from build123d import *

# Parameters (mm, degrees)
BOSS_EXTRUDE1_DEPTH = 7
SKETCH2_R           = 2.5
CUT_EXTRUDE1_DEPTH  = 14


with BuildPart() as part:
    # Sketch1 → Boss-Extrude1 (new, symmetric)
    with BuildSketch(Plane(origin=(0, 0, 0), x_dir=(1, 0, 0), z_dir=(0, 1, 0))):
        Polygon((7, 1.5), (-7, 1.5), (-4, -1.5), (4, -1.5), align=None)
    extrude(amount=BOSS_EXTRUDE1_DEPTH, both=True)

    # Sketch2 → Cut-Extrude1 (cut)
    with BuildSketch(Plane(origin=(0, 0, -1.5), x_dir=(-1, 0, 0), z_dir=(0, 0, -1))):
        Circle(SKETCH2_R)
    extrude(amount=-CUT_EXTRUDE1_DEPTH, mode=Mode.SUBTRACT)


solid = part.part
Design review of the part built by this model. Coordinates are the model's own, in mm. Coordinates: 2 decimals unless noted, no trailing zeros. Order: outer loops, then holes, each group sorted by start corner. A loop starts at its lowest first (then second) coordinate and runs counter-clockwise, first axis right, second up. Notation, with made-up numbers: (57, 32.25) -> (113, 32.25) arc R10 cw to (113, 37.25) -> close; hole circle Ø11 at (26.25, 79.25). An arc over 180 degrees is marked (long way). Use one line per item in the form item = value. Start each with the question number.
(1) Add section D-D on y = 5. State the section outline as (x, z) points.
(2) Insertion check: pin 1 (1 mm diameter, centred on y = 5.5, z = 1, fed in from -X). The pin has a flat end and moves straight along its axis. Give the tip position at first contact, or say it passes through.
(3) For probe 1 along Y at (x, z) = (0, -0.5); probe 2 along Y at (x, z) = (-1, 0.55); probe 3 along Z at (x, y) = (-5, -6), list the stretches that pass through material, from the lowest coordinate up.
(4) The part is to be moulded in two halves that separate along X. For faces 1 (the flat face through (-5.5, 0.1, 0)), 2 (the cylindrical face through (0.54, -2.44, -0.02)), 3 (the flat face through (0, 7, 0)), say which applies: +X half, -X half, draft (parallel to the pull), parting line (faces both ways), or undercut.
(5) Add section C-C on z = 0.6. State the section outline as (x, y) points.
(6) Add section B-B on y = 0. State the section outline as (x, z) points, plus the area to 3 significant figures.
(7) Add section A-A on x = -2. State the section outline as (y, z) points, plus the area to 3 significant figures.
Answer block:
q1.outline = (-7, -1.5) -> (7, -1.5) -> (4, 1.5) -> (-4, 1.5) -> close
q2.pin_1 = -5
q3.probe_1 = -7 to -2.5, 2.5 to 7
q3.probe_2 = -7 to -2.29, 2.29 to 7
q3.probe_3 = -1.5 to 0.5
q4.face_1 = -X half
q4.face_2 = undercut
q4.face_3 = draft
q5.outline = (-4.9, -7) -> (4.9, -7) -> (4.9, 7) -> (-4.9, 7) -> close; hole circle Ø5 at (0, 0)
q6.outline = (-7, -1.5) -> (-2.5, -1.5) -> (-2.5, 1.5) -> (-4, 1.5) -> close; (2.5, -1.5) -> (7, -1.5) -> (4, 1.5) -> (2.5, 1.5) -> close
q6.area = 18.0 mm²
q7.outline = (-7, -1.5) -> (-1.5, -1.5) -> (-1.5, 1.5) -> (-7, 1.5) -> close; (1.5, -1.5) -> (7, -1.5) -> (7, 1.5) -> (1.5, 1.5) -> close
q7.area = 33.0 mm²
